Source: CAD feature listing. Evaluate the final solid. Frame: model axes, mm. A direction names the side the tool comes from. Coordinates: 2 decimals unless noted, no trailing zeros. Write each loop counter-clockwise with the first axis right and the second up, starting at its lowest first coordinate (ties: lowest second). Pieces come first, ordered by that corner, then holes. Notation, with made-up numbers: (16, 56.5) -> (66, 56.5) arc R16 cw to (66, 74.5) -> close; hole circle Ø9 at (86, -38). An arc over 180 degrees is marked (long way). One line per item, written item: value. Start each with the question number.
1. Line query: line 1 (Z direction, x = -2, y = 7.75); line 2 (X direction, y = 4.25, z = -3); line 3 (Y direction, x = -6.5, z = 4). Output: solid intervals per line, ascending.
2. Section query A-A, the plane y = 2.75. Output: boundary loops of the cut face in (x, z).
3. Section query D-D, the plane x = -5. Output: boundary loops of the cut face in (y, z), and give its area (3 significant figures).
4. Section query B-B, the plane x = -0.75. Output: boundary loops of the cut face in (y, z).
5. Access query for faces 4 (the flat face through (1.511, 3, 0)), 5 (the flat face through (-5, -1, -7.5)), 6 (the cylindrical face through (2.656, 8.949, -31.598)). Directions: +Z, -Z, +X, -X, +Y, -Y. A direction counts if a zero-diameter tool reaches every point of the face in a straight line with its end or side. Return the directions, or none.
6. First-contact query: P1, Ø3, axis at x = -8.5, z = -21, coming from the -Y side. Flat tip, straight axial feed; report the tip coordinate or a pass-through.
7. Mould query, pull axis Z, two halves, no side actions, for faces 1 (the flat face through (-5, -2.079, 0)), 2 (the cylindrical face through (-2.7, 8.95, -23.25)), 3 (the flat face through (-5, 9, -32.5)). Classes: released by +Z, released by -Z, zero draft, split by the parting line, or undercut.
8. Section query C-C, the plane z = 4.5. Output: boundary loops of the cut face in (x, y), and give its area (3 significant figures).
from build123d import *

# Parameters (mm, degrees)
F0_W     = 17.6
F0_H     = 9
F0_W_2   = 13.6
F0_H_2   = 6.4
F1_DEPTH = 7.5
F2_W     = 17.6
F2_H     = 15
F2_H_2   = 25
F3_DEPTH = 4
F4_SIZE  = 0.6
F5_D     = 4.6
F5_DEPTH = 10
F5_TIP   = 1.3819794238
F6_R     = 3


# Not quite as in the source:
# - a feature names something its author has since deleted; it is built from what else it names


with BuildPart() as f1:
    # F0 (on Top) → F1 (new body, symmetric)
    with BuildSketch(Plane.XY):
        with Locations((-5.2887722373, 2.4212898893)):
            Rectangle(F0_W, F0_H)
        with Locations((-5.2887722373, 3.1212898893)):
            Rectangle(F0_W_2, F0_H_2, mode=Mode.SUBTRACT)
    extrude(amount=F1_DEPTH, both=True)

    # F2 (on face) → F3 (join)
    with BuildSketch(Plane(origin=(0, 6.9212898893, 0), x_dir=(-1, 0, 0), z_dir=(0, 1, 0))):
        with Locations((5.2887722373, 0)):
            Rectangle(F2_W, F2_H)
        with Locations((5.2887722373, -20)):
            Rectangle(F2_W, F2_H_2)
    extrude(amount=F3_DEPTH)

    # F4
    f4_edges = [f1.edges().sort_by_distance(p)[0] for p in [
        (-5.288772, 6.32129, 7.5),
        (1.511228, 3.12129, 7.5),
        (-12.088772, 3.12129, 7.5),
        (-5.288772, -0.07871, 7.5),
    ]]
    chamfer(f4_edges, length=F4_SIZE)

    # F5
    with Locations(Plane(origin=(0, 6.9212898893, 0), x_dir=(-1, 0, 0), z_dir=(0, -1, 0))):
        with Locations((2.2041960619, 25.4963655025), (2.2041960619, 13.4963655025)):
            Hole(F5_D / 2, depth=F5_DEPTH)
            with Locations((0, 0, -(F5_DEPTH + F5_TIP / 2))):  # 118° drill point
                Cone(0, F5_D / 2, F5_TIP, mode=Mode.SUBTRACT)

    # F6
    f6_edges = [f1.edges().sort_by_distance(p)[0] for p in [
        (3.511228, 8.92129, -32.5),
        (-14.088772, 8.92129, -32.5),
    ]]
    fillet(f6_edges, radius=F6_R)


solid = f1.part
Computed values:
1. line 1: z = -32.5 to -27.79, -23.21 to -15.79, -11.21 to 7.5
1. line 2: x = -14.09 to -12.09, 1.51 to 3.51
1. line 3: y = -2.08 to -0.08, 6.32 to 10.92
2. outline: (-14.09, -7.5) -> (-12.09, -7.5) -> (-12.09, 6.9) -> (-12.69, 7.5) -> (-14.09, 7.5) -> close; (1.51, -7.5) -> (3.51, -7.5) -> (3.51, 7.5) -> (2.11, 7.5) -> (1.51, 6.9) -> close
3. outline: (-2.08, -7.5) -> (-0.08, -7.5) -> (-0.08, 6.9) -> (-0.68, 7.5) -> (-2.08, 7.5) -> close; (6.32, -7.5) -> (6.92, -7.5) -> (6.92, -32.5) -> (10.92, -32.5) -> (10.92, 7.5) -> (6.92, 7.5) -> (6.32, 6.9) -> close
3. area: 199 mm²
4. outline: (-2.08, -7.5) -> (-0.08, -7.5) -> (-0.08, 6.9) -> (-0.68, 7.5) -> (-2.08, 7.5) -> close; (6.32, -7.5) -> (6.92, -7.5) -> (6.92, -11.71) -> (10.92, -11.71) -> (10.92, 7.5) -> (6.92, 7.5) -> (6.32, 6.9) -> close; (6.92, -32.5) -> (10.92, -32.5) -> (10.92, -27.28) -> (6.92, -27.28) -> close; (6.92, -23.71) -> (10.92, -23.71) -> (10.92, -15.28) -> (6.92, -15.28) -> close
5. face 4: +Z, -Z
5. face 5: -Z, +X, -X, -Y
5. face 6: -Z, +X, +Y, -Y
6. P1: stops at y = 6.92
7. face 1: zero draft
7. face 2: undercut
7. face 3: released by -Z
8. outline: (-14.09, -2.08) -> (3.51, -2.08) -> (3.51, 10.92) -> (-14.09, 10.92) -> close; hole (-12.09, -0.08) -> (1.51, -0.08) -> (1.51, 6.32) -> (-12.09, 6.32) -> close
8. area: 142 mm²
